from build123d import *

# Parameters (mm, degrees)
F0_W      = 32
F0_H      = 32
F1_DEPTH  = 40
F2_R      = 4.7625
F3_DEPTH  = 10
F4_R      = 4.7625
F5_DEPTH  = 10
F6_R      = 11.1
F7_DEPTH  = 3
F8_R      = 11.05
F9_DEPTH  = 3
F10_R     = 5.1
F11_DEPTH = 80.001
F12_R     = 6.7625
F12_R_2   = 4.7625
F13_DEPTH = 6
F14_R     = 6.7625
F14_R_2   = 4.7625
F15_DEPTH = 6


with BuildPart() as f1:
    # F0 (on Top) → F1 (new body, symmetric)
    with BuildSketch(Plane.XY):
        Rectangle(F0_W, F0_H)
    extrude(amount=F1_DEPTH, both=True)

    # F2 (on face) → F3 (cut)
    with BuildSketch(Plane.YZ.offset(16)):
        with Locations((0, 21.5)):
            Circle(F2_R)
        with Locations((0, -21.5)):
            Circle(F2_R)
    extrude(amount=-F3_DEPTH, mode=Mode.SUBTRACT)

    # F4 (on face) → F5 (cut)
    with BuildSketch(Plane.XZ.offset(16)):
        with Locations((0, 21.5)):
            Circle(F4_R)
        with Locations((0, -21.5)):
            Circle(F4_R)
    extrude(amount=-F5_DEPTH, mode=Mode.SUBTRACT)

    # F6 (on face) → F7 (cut)
    with BuildSketch(Plane.XY.offset(40)):
        Circle(F6_R)
    extrude(amount=-F7_DEPTH, mode=Mode.SUBTRACT)

    # F8 (on face) → F9 (cut)
    with BuildSketch(Plane(origin=(0, 0, -40), x_dir=(1, 0, 0), z_dir=(0, 0, -1))):
        Circle(F8_R)
    extrude(amount=-F9_DEPTH, mode=Mode.SUBTRACT)

    # F10 (on face) → F11 (cut, through all)
    with BuildSketch(Plane(origin=(0, 0, -40), x_dir=(1, 0, 0), z_dir=(0, 0, -1))):
        Circle(F10_R)
    extrude(amount=-F11_DEPTH, mode=Mode.SUBTRACT)

    # F12 (on face) → F13 (join)
    with BuildSketch(Plane.YZ.offset(16)):
        with Locations((0, 21.5)):
            Circle(F12_R)
        with Locations((0, 21.5)):
            Circle(F12_R_2, mode=Mode.SUBTRACT)
        with Locations((0, -21.5)):
            Circle(F12_R)
        with Locations((0, -21.5)):
            Circle(F12_R_2, mode=Mode.SUBTRACT)
    extrude(amount=F13_DEPTH)

    # F14 (on face) → F15 (join)
    with BuildSketch(Plane.XZ.offset(16)):
        with Locations((0, 21.5)):
            Circle(F14_R)
        with Locations((0, 21.5)):
            Circle(F14_R_2, mode=Mode.SUBTRACT)
        with Locations((0, -21.5)):
            Circle(F14_R)
        with Locations((0, -21.5)):
            Circle(F14_R_2, mode=Mode.SUBTRACT)
    extrude(amount=F15_DEPTH)


solid = f1.part
Verification items for the finished model (mm, model axes). A direction names the side the tool comes from. Give positions to 0.01 mm unless a question says otherwise; leave off trailing zeros. Write each loop counter-clockwise with the first axis right and the second up, starting at its lowest first coordinate (ties: lowest second). Pieces come first, ordered by that corner, then holes. Notation, with made-up numbers: M 67,42.25 L 73,42.25 A30 ccw 73,75.25 Z; hole C -22.75,68 d2. An arc over 180 degrees is marked long. Use CSV: the item, a comma, the result in double quotes.
1) Cross-section at D-D (z = -32.5). Enter the section's corners in (x, y), plus the area to 3 significant figures.
Final values:
outline,"M -16,-16 L 16,-16 L 16,16 L -16,16 Z; hole C 0,0 d10.2"
area,"942 mm²"
2) Release check for a two-part mould opening along Z. For faces 6 (the face through (22, -5, -23)), 7 (the face through (-4, 11, 40)), 8 (the face through (0, -6, 22)) record: released by +Z, released by -Z, zero draft, split by the parting line, or undercut.
Final values:
face 6,"zero draft"
face 7,"released by +Z"
face 8,"undercut"
3) Cross-section at B-B (z = -21.5). Enter the section's corners in (x, y), plus the area to 3 significant figures.
Final values:
outline,"M -16,-16 L -6.76,-16 L -6.76,-22 L -4.76,-22 L -4.76,-6 L 4.76,-6 L 4.76,-22 L 6.76,-22 L 6.76,-16 L 16,-16 L 16,-6.76 L 22,-6.76 L 22,-4.76 L 6,-4.76 L 6,4.76 L 22,4.76 L 22,6.76 L 16,6.76 L 16,16 L -16,16 Z; hole C 0,0 d10.2"
area,"800 mm²"
4) Access from +Z, -Z, +X, -X, +Y, -Y to the whole of each face (thin tool, end or side, straight path). Record for faces 1 (the face through (-5.37, -18.96, 17.39)), 2 (the face through (5, 2, -37)), 3 (the face through (-5, -22, -23)), 4 (the face through (5, -2, 37)), 5 (the face through (13.89, -1.03, -26.15)).
Final values:
face 1,"-Y"
face 2,"-Z"
face 3,"+Z, -Z, +X, -X, -Y"
face 4,"+Z"
face 5,"+X"
5) Material ranges on line 1 along Z through (x, y) = (0, -14); line 2 along Z through (x, y) = (10.5, 0); line 3 along Y through (x, z) = (0, 2), recorded low to high.
Final values:
line 1,"-40 to -26.26, -16.74 to 16.74, 26.26 to 40"
line 2,"-37 to -26.26, -16.74 to 16.74, 26.26 to 37"
line 3,"-16 to -5.1, 5.1 to 16"
6) Go/stop test with flat-tipped pins: pin 1 Ø4 at (x, y) = (-1.5, 6) entering from +Z; pin 2 Ø12 at (x, z) = (-1, 30.5) entering from -Y; pin 3 Ø13.5 at (x, y) = (0, 0) entering from -Z; pin 4 Ø4 at (x, z) = (4.5, 4.5) entering from -Y. Record where each tip stops, or that it passes through.
Final values:
pin 1,"z = 37"
pin 2,"y = -22"
pin 3,"z = -37"
pin 4,"y = -16"
